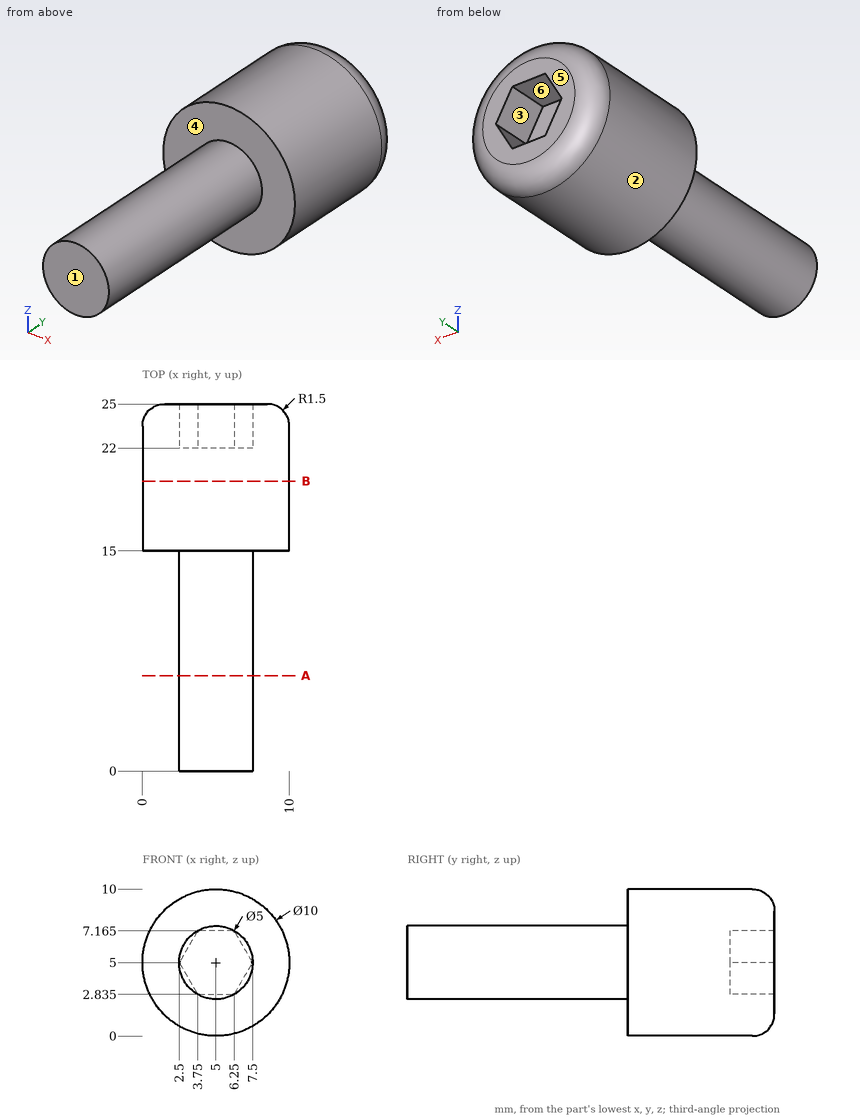
The drawing under review shows one solid part. Ordinate dimensions are in mm from its lowest x, y, z. A direction names the side the tool comes from. Round coordinates to 2 decimals unless told otherwise and drop trailing zeros. Loops run counter-clockwise (first coordinate to the right, second up) from the corner with the lowest first, then second, coordinate; pieces in that order, holes last. Notation, with made-up numbers: M 86,-21 L 121,-21 A26 cw 121,17 Z; hole C -15,-7 d7. An arc over 180 degrees is marked long. Answer as CSV lines item,"result". Start each with the question number.
Item 1: For the marked faces 4, 5 and 6, list the 3-axis set-ups (+Z, -Z, +X, -X, +Y, -Y) from which the entire face can be reached by the end or side of a thin tool; tool diameter is ignored.
Item 2: Consider section B-B (y = 19.75). Write out the cut boundary in (x, z).
Item 3: Consider section A-A (y = 6.5). Write out the cut boundary in (x, z), then the cut area to 3 significant figures.
Item 4: Mouldability with a two-part tool opening along X and no side actions: class the marked faces 1, 2 and 3 as released by +X, released by -X, zero draft, split by the parting line, or undercut.
Item 5: Wall thickness on line 1 (Z direction, x = 3.25, y = 22.25); line 2 (X direction, y = 22.5, z = 3.25); line 3 (X direction, y = 13, z = 5.5): over which ranges is each line inside the solid? List them lowest first. Write a range as [from, to].
Item 6: Insertion check: P1, Ø1.2, axis at x = 4.5, y = 24, coming from the -Z side; P2, Ø1, axis at y = 9, z = 5, coming from the +X side; P3, Ø1.5, axis at x = 8, y = 6, coming from the -Z side. Each pin has a flat end and moves straight along its axis. Give the tip position at first contact, or say it passes through.
Answer:
1,face 4,"-Y"
1,face 5,"+Z, -Z, +X, -X, +Y"
1,face 6,"+Y"
2,outline,"C 5,5 d10"
3,outline,"C 5,5 d5"
3,area,"19.6 mm^2"
4,face 1,"zero draft"
4,face 2,"split by the parting line"
4,face 3,"undercut"
5,line 1,"z = [0.32, 3.7], [6.3, 9.68]"
5,line 2,"x = [0.32, 3.51], [6.49, 9.68]"
5,line 3,"x = [2.55, 7.45]"
6,P1,"stops at z = 0"
6,P2,"stops at x = 7.5"
6,P3,"stops at z = 3.91"
